Design review of the part built by this model. Coordinates are the model's own, in mm. A direction names the side the tool comes from. Coordinates: 2 decimals unless noted, no trailing zeros. Loops run counter-clockwise (first coordinate to the right, second up) from the corner with the lowest first, then second, coordinate; pieces in that order, holes last. Notation, with made-up numbers: (20, 8) - (43, 8) arc R24 ccw to (43, 33) - close; hole circle Ø9 at (-21.5, 84.25). An arc over 180 degrees is marked (long way). Return JSON: item names as keys, results as strings. Group by question number.
from build123d import *
from OCP.BRepFilletAPI import BRepFilletAPI_MakeChamfer
from build123d.topology import SkipClean

# Parameters (mm, degrees)
SKETCH1_W           = 40
SKETCH1_H           = 28.5
SKETCH1_R           = 3
BOSS_EXTRUDE1_DEPTH = 5
SKETCH2_W           = 32.5
SKETCH2_H           = 51
CUT_EXTRUDE1_DEPTH  = 10
SKETCH3_W           = 137.62708118
SKETCH3_H           = 29.533708408
CUT_EXTRUDE2_DEPTH  = 10
BOSS_EXTRUDE2_START = 8.5
SKETCH4_R           = 3
BOSS_EXTRUDE2_DEPTH = 8.5
FILLET1_R           = 5
SKETCH5_W           = 8
SKETCH5_H           = 8
SKETCH5_W_2         = 35
SKETCH5_H_2         = 10
CUT_EXTRUDE3_DEPTH  = 13.5
BOSS_EXTRUDE6_START = -13.5
SKETCH6_W           = 3
SKETCH6_H           = 5
BOSS_EXTRUDE6_DEPTH = 13.5
CUT_EXTRUDE4_START  = -10
SKETCH7_R           = 5.5
SKETCH7_R_2         = 3
CUT_EXTRUDE4_DEPTH  = 10
CHAMFER1_SIZE       = 5
CHAMFER1_SIZE_2     = 2.886751346
CHAMFER2_SIZE       = 5.196152423
CHAMFER2_SIZE_2     = 3


# Some blends are built 0.0001 mm under size
with BuildPart() as part:
    # Sketch1 → Boss-Extrude1 (new body)
    with BuildSketch(Plane(origin=(0, 0, 0), x_dir=(1, 0, 0), z_dir=(0, 1, 0))):
        with BuildLine():
            Line((-31.5, 11), (-31.5, -11))
            Line((-31.5, -11), (-56.629054395, -18.053769655))
            add(Edge.make_bspline(
                [(-56.629054395, -18.053769655), (-58.486129852, -20.409089771), (-60, -22.885467918)],
                knots=[0.137055219, 0.137055219, 0.137055219, 0.224914017, 0.224914017, 0.224914017], degree=2))
            Line((-60, -22.885467918), (-60, -76))
            Line((-60, -76), (-27.5, -76))
            Line((-27.5, -76), (-27.5, -81))
            Line((-27.5, -81), (27.5, -81))
            Line((27.5, -81), (27.5, -76))
            Line((27.5, -76), (60, -76))
            Line((60, -76), (60, -22.885467918))
            add(Edge.make_bspline(
                [(56.629054395, -18.053769655), (58.486129852, -20.409089771), (60, -22.885467918)],
                knots=[0.137055219, 0.137055219, 0.137055219, 0.224914017, 0.224914017, 0.224914017], degree=2))
            Line((56.629054395, -18.053769655), (31.5, -11))
            Line((31.5, -11), (31.5, 11))
            Line((31.5, 11), (5.25, 11))
            Line((5.25, 11), (5.25, -11))
            Line((5.25, -11), (-5.25, -11))
            Line((-5.25, -11), (-5.25, 11))
            Line((-5.25, 11), (-31.5, 11))
        make_face()
        with Locations((0, -61.75)):
            Rectangle(SKETCH1_W, SKETCH1_H, mode=Mode.SUBTRACT)
        with Locations(Location((-20, 0, 0), (0, 0, 270))):
            Circle(SKETCH1_R, mode=Mode.SUBTRACT)
        with Locations(Location((20, 0, 0), (0, 0, 270))):
            Circle(SKETCH1_R, mode=Mode.SUBTRACT)
    extrude(amount=BOSS_EXTRUDE1_DEPTH)

    # Sketch2 → Cut-Extrude1 (cut)
    with BuildSketch(Plane(origin=(0, 5, 0), x_dir=(1, 0, 0), z_dir=(0, 1, 0))):
        with Locations((-37.75, -47.5)):
            Rectangle(SKETCH2_W, SKETCH2_H)
        with Locations((37.75, -47.5)):
            Rectangle(SKETCH2_W, SKETCH2_H)
    extrude(amount=-CUT_EXTRUDE1_DEPTH, mode=Mode.SUBTRACT)

    # Sketch3 → Cut-Extrude2 (cut)
    with BuildSketch(Plane(origin=(0, 5, 0), x_dir=(1, 0, 0), z_dir=(0, 1, 0))):
        with Locations((-0.764574483, 21.766854204)):
            Rectangle(SKETCH3_W, SKETCH3_H)
    extrude(amount=-CUT_EXTRUDE2_DEPTH, mode=Mode.SUBTRACT)

    # Sketch4 → Boss-Extrude2 (add)
    # profile 1 of 3: a face of its own
    with SkipClean():  # the faces are left unmerged after this step: merging them gives an invalid solid
        with BuildSketch(Plane.XZ.offset(BOSS_EXTRUDE2_START)):
            Polygon((-41.5, 20.807017544), (-41.5, 13.807017544), (-31.5, 11), (-31.5, -7), (-5.25, -7), (-5.25, 11), (5.25, 11), (5.25, -7), (31.5, -7), (31.5, 11), (41.5, 13.807017544), (41.5, 20.807017544), (21.5, 20.807017544), (21.5, 44.307017544), (-21.5, 44.307017544), (-21.5, 20.807017544), align=None)
            with Locations(Location((-20, 0, 0), (0, 0, 270))):
                Circle(SKETCH4_R, mode=Mode.SUBTRACT)
            with Locations(Location((20, 0, 0), (0, 0, 270))):
                Circle(SKETCH4_R, mode=Mode.SUBTRACT)
        # profile 2 of 3: a face of its own
        with BuildSketch(Plane.XZ.offset(BOSS_EXTRUDE2_START)):
            Polygon((-60, 61), (-54, 61), (-54, 73), (-21.5, 73), (-21.5, 81), (-27.5, 81), (-27.5, 76), (-60, 76), align=None)
        # profile 3 of 3: a face of its own
        with BuildSketch(Plane.XZ.offset(BOSS_EXTRUDE2_START)):
            Polygon((27.5, 81), (21.5, 81), (21.5, 73), (54, 73), (54, 61), (60, 61), (59.999999958, 73), (60, 76), (27.5, 76), align=None)
        extrude(amount=-BOSS_EXTRUDE2_DEPTH)

    # Fillet1
    fillet1_edges = [part.edges().sort_by_distance(p)[0] for p in [
        (60, -4.25, 76),
        (-60, -4.25, 76),
    ]]
    fillet(fillet1_edges, radius=FILLET1_R)

    # Sketch5 → Cut-Extrude3 (cut)
    with SkipClean():  # the faces are left unmerged after this step: merging them gives an invalid solid
        with BuildSketch(Plane(origin=(0, 5, 0), x_dir=(1, 0, 0), z_dir=(0, 1, 0))):
            with Locations((0, -18)):
                Rectangle(SKETCH5_W, SKETCH5_H)
            with Locations((0, -26)):
                Rectangle(SKETCH5_W_2, SKETCH5_H)
            with Locations((0, -35)):
                Rectangle(SKETCH5_W, SKETCH5_H_2)
        extrude(amount=-CUT_EXTRUDE3_DEPTH, mode=Mode.SUBTRACT)

    # Sketch6 → Boss-Extrude6 (add)
    with SkipClean():  # the faces are left unmerged after this step: merging them gives an invalid solid
        with BuildSketch(Plane(origin=(0, 5, 0), x_dir=(1, 0, 0), z_dir=(0, 1, 0)).offset(BOSS_EXTRUDE6_START)):
            with Locations((-52.5, -70.5)):
                Rectangle(SKETCH6_W, SKETCH6_H)
            with Locations((-23, -70.5)):
                Rectangle(SKETCH6_W, SKETCH6_H)
            Polygon((-21.5, -73), (-24.5, -73), (-27.5, -73), (-27.5, -76), (-21.5, -76), align=None)
            with Locations((23, -70.5)):
                Rectangle(SKETCH6_W, SKETCH6_H)
            Polygon((27.5, -73), (24.5, -73), (21.5, -73), (21.5, -76), (27.5, -76), align=None)
            with Locations((52.5, -70.5)):
                Rectangle(SKETCH6_W, SKETCH6_H)
        extrude(amount=BOSS_EXTRUDE6_DEPTH)

    # Sketch7 → Cut-Extrude4 (cut)
    # profile 1 of 2: a face of its own
    with BuildSketch(Plane(origin=(0, 5, 0), x_dir=(1, 0, 0), z_dir=(0, 1, 0)).offset(CUT_EXTRUDE4_START)):
        with Locations(Location((-20, 0, 0), (0, 0, 270))):
            Circle(SKETCH7_R)
        with Locations(Location((-20, 0, 0), (0, 0, 90))):
            Circle(SKETCH7_R_2, mode=Mode.SUBTRACT)
    # profile 2 of 2: a face of its own
    with BuildSketch(Plane(origin=(0, 5, 0), x_dir=(1, 0, 0), z_dir=(0, 1, 0)).offset(CUT_EXTRUDE4_START)):
        with Locations(Location((20, 0, 0), (0, 0, 270))):
            Circle(SKETCH7_R)
        with Locations(Location((20, 0, 0), (0, 0, 90))):
            Circle(SKETCH7_R_2, mode=Mode.SUBTRACT)
    extrude(amount=CUT_EXTRUDE4_DEPTH, mode=Mode.SUBTRACT)

    # Chamfer1
    chamfer1_edges_1 = [part.edges().sort_by_distance(p)[0] for p in [
        (51, -1.75, 68),
    ]]
    chamfer1_side_1 = [part.faces().sort_by_distance(p)[0] for p in [
        (51, -1.75, 68.057735027),
    ]]
    chamfer1_edges_2 = [part.edges().sort_by_distance(p)[0] for p in [
        (-24.5, -1.75, 68),
    ]]
    chamfer1_side_2 = [part.faces().sort_by_distance(p)[0] for p in [
        (-24.5, -1.75, 68.057735027),
    ]]
    chamfer1 = BRepFilletAPI_MakeChamfer(part.part.solid().wrapped)
    for e in chamfer1_edges_1:
        chamfer1.Add(CHAMFER1_SIZE - 0.0001, CHAMFER1_SIZE_2 - 0.0001, e.wrapped, chamfer1_side_1[0].wrapped)
    for e in chamfer1_edges_2:
        chamfer1.Add(CHAMFER1_SIZE - 0.0001, CHAMFER1_SIZE_2 - 0.0001, e.wrapped, chamfer1_side_2[0].wrapped)
    add(Compound.cast(chamfer1.Shape()), mode=Mode.REPLACE)  # a hair under: the kernel refuses the full size

    # Chamfer2
    # the kernel refuses this chamfer: 5.196152423, 3 mm, written as the material it takes off along each edge
    with BuildSketch(Plane(origin=(-51, -21.942891912, 68), x_dir=(0.01932676561269968, 0, 0.9998132206222079), z_dir=(0, 1, 0))) as chamfer2_piece_1_section:
        Polygon((CHAMFER2_SIZE * 0.999813220566, -CHAMFER2_SIZE * 0.0193267656116), (-CHAMFER2_SIZE_2 * 0.0193267656127, -CHAMFER2_SIZE_2 * 0.999813220622), (0, 0), align=None)
    chamfer2_piece_1 = extrude(amount=40.385783824, mode=Mode.PRIVATE)
    chamfer2_piece_1 = split(chamfer2_piece_1, bisect_by=Plane(origin=(-51.966537061, -1.75, 73), z_dir=(0, 0, -1)), keep=Keep.TOP, mode=Mode.PRIVATE)
    chamfer2_piece_1 = split(chamfer2_piece_1, bisect_by=Plane(origin=(-54, -1.75, 69.717275258), z_dir=(1, 0, 0)), keep=Keep.TOP, mode=Mode.PRIVATE)
    add(chamfer2_piece_1, mode=Mode.SUBTRACT)
    with BuildSketch(Plane(origin=(24.5, -21.942891912, 68), x_dir=(0.019326765612701, 0, 0.9998132206222079), z_dir=(0, 1, 0))) as chamfer2_piece_2_section:
        Polygon((CHAMFER2_SIZE * 0.999813220566, -CHAMFER2_SIZE * 0.0193267656116), (-CHAMFER2_SIZE_2 * 0.0193267656127, -CHAMFER2_SIZE_2 * 0.999813220622), (0, 0), align=None)
    chamfer2_piece_2 = extrude(amount=40.385783824, mode=Mode.PRIVATE)
    chamfer2_piece_2 = split(chamfer2_piece_2, bisect_by=Plane(origin=(23.533462939, -1.75, 73), z_dir=(0, 0, -1)), keep=Keep.TOP, mode=Mode.PRIVATE)
    add(chamfer2_piece_2, mode=Mode.SUBTRACT)


solid = part.part
Item 1: Add section D-D (x = -36). State the section outline as (y, z) points, then the cut area to 3 significant figures.
Item 2: Add section C-C (y = -1.25). Give the number of separate pieces and of enclosed holes in the cut face, then the cut area to 3 significant figures.
Item 3: For P1, Ø4, axis at x = 9.5, y = -4, coming from the +Z side; P2, Ø4, axis at x = 37.5, y = -0.5, coming from the -Z side; P3, Ø3, axis at y = 0.5, z = 20.5, coming from the -X side, all flat-tipped, find the tip position at first contact; note any pin that passes through.
Item 4: Add section B-B (z = 0). State the section outline as (x, y) points, then the cut area to 3 significant figures.
Item 5: Draft analysis for pull direction Z (two halves, no side actions). For faces 4 (the face through (-57, -4, 61)), 5 (the face through (-31.5, -2, 2)), 6 (the face through (-4, -2, 35)), state which applies: pulls with the +Z half, pulls with the -Z half, needs draft (parallel to the pull), parting line crosses it, or undercut.
Item 6: Add section A-A (x = 9). State the section outline as (y, z) points, then the cut area to 3 significant figures.
Item 7: For faces 1 (the face through (0, -2, 40)), 2 (the face through (57, -4, 61)), 3 (the face through (5.25, -2, 2)), list the 3-axis set-ups (+Z, -Z, +X, -X, +Y, -Y) from which the entire face can be reached by the end or side of a thin tool; tool diameter is ignored.
Item 8: To check wall thickness, follow line 1 (X direction, y = 0.75, z = 0); line 2 (X direction, y = 3, z = 26.5); line 3 (Z direction, x = -31, y = 1.25). State the ranges of each line that lie inside material, in increasing order. Write a range as from..to.
Answers below:
{
 "1": {"outline": "(-8.5, 12.26) - (5, 12.26) - (5, 22) - (0, 22) - (0, 20.81) - (-8.5, 20.81) - close; (-8.5, 73) - (5, 73) - (5, 76) - (-8.5, 76) - close", "area": "162 mm^2"},
 "2": {"separate pieces": "3", "enclosed holes": "3", "area": "2,580 mm^2"},
 "3": {"P1": "stops at z = 44.31", "P2": "stops at z = 12.12", "P3": "stops at x = -59.45"},
 "4": {"outline": "(-31.5, -8.5) - (-23, -8.5) - (-23, -5) - (-25.5, -5) - (-25.5, 5) - (-31.5, 5) - close; (-17, -8.5) - (-5.25, -8.5) - (-5.25, 5) - (-14.5, 5) - (-14.5, -5) - (-17, -5) - close; (5.25, -8.5) - (17, -8.5) - (17, -5) - (14.5, -5) - (14.5, 5) - (5.25, 5) - close; (23, -8.5) - (31.5, -8.5) - (31.5, 5) - (25.5, 5) - (25.5, -5) - (23, -5) - close", "area": "447 mm^2"},
 "5": {"face 4": "pulls with the -Z half", "face 5": "needs draft", "face 6": "undercut"},
 "6": {"outline": "(-8.5, -7) - (5, -7) - (5, 22) - (-8.5, 22) - close; (-8.5, 30) - (5, 30) - (5, 47.5) - (0, 47.5) - (0, 44.31) - (-8.5, 44.31) - close; (0, 76) - (5, 76) - (5, 81) - (0, 81) - close", "area": "626 mm^2"},
 "7": {"face 1": "+Y, -Y", "face 2": "-Z, +X, -X, -Y", "face 3": "-Z, +Y, -Y"},
 "8": {"line 1": "x = -31.5..-25.5, -14.5..-5.25, 5.25..14.5, 25.5..31.5", "line 2": "x = -60..-54, -21.5..-17.5, 17.5..21.5, 54..60", "line 3": "z = -7..22, 73..76"}
}
